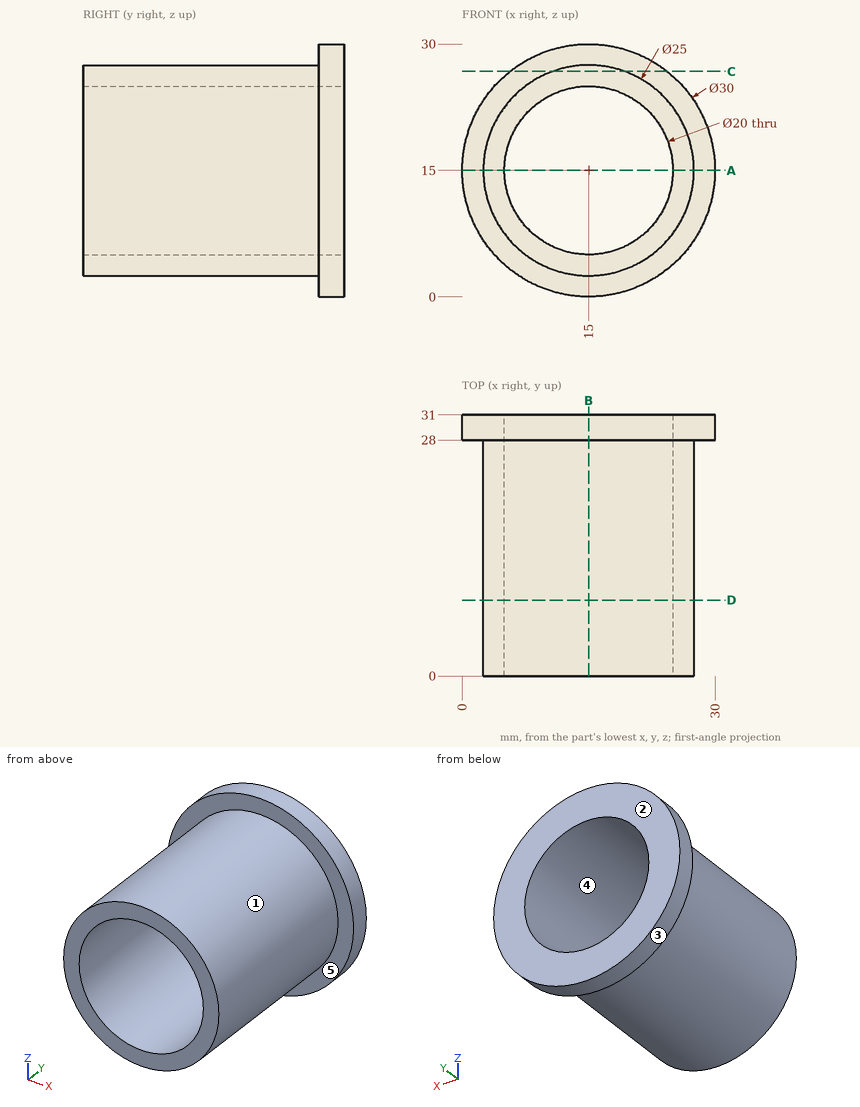
Answer from the drawing. Dimensions are ordinates in mm from the lowest x, y and z of the part. A direction names the side the tool comes from. Round coordinates to 2 decimals unless told otherwise and drop trailing zeros. Loops run counter-clockwise (first coordinate to the right, second up) from the corner with the lowest first, then second, coordinate; pieces in that order, holes last.
Q1. Section B-B on x = 15 is taken. Write down the section's boundary in (y, z), and give its area (3 significant figures).
Q2. Section D-D on y = 9 is taken. Write down the section's boundary in (x, z), and give its area (3 significant figures).
Q3. Section A-A on z = 15 is taken. Write down the section's boundary in (x, y).
Q4. Section C-C on z = 26.75 is taken. Write down the section's boundary in (x, y), and give its area (3 significant figures).
Q5. Which of the six approach directions +Z, -Z, +X, -X, +Y, -Y give full straight-line access (tool end or side, diameter ignored) to the marked faces 1 and 2?
Q6. Determine the mould class of the marked faces 3, 4 and 5 for opening direction Z: released by +Z, released by -Z, zero draft, split by the parting line, or undercut.
Q7. Consider probe 1 along Z at (x, y) = (15, 8.5); probe 2 along Y at (x, z) = (21.25, 2.5); probe 3 along X at (y, z) = (28.5, 21.75). Determine where each line is inside the solid, lowest interval first.
Q8. Each of these flat-tipped pins is pushed along its axis until it touches: pin 1 (10 mm diameter, centred on x = 21, y = 26.5, fed in from -Z); pin 2 (10 mm diameter, centred on y = 10.5, z = 9, fed in from -X); pin 3 (1.5 mm diameter, centred on y = 17, z = 6.5, fed in from -X); pin 4 (6 mm diameter, centred on x = 18.5, z = 23.5, fed in from -Y). Where does it stop, or does it pass through?
Output:
1. outline: (0, 2.5) - (28, 2.5) - (28, 0) - (31, 0) - (31, 5) - (0, 5) - close; (0, 25) - (31, 25) - (31, 30) - (28, 30) - (28, 27.5) - (0, 27.5) - close
1. area: 170 mm2
2. outline: circle Ø25 at (15, 15); hole circle Ø20 at (15, 15)
2. area: 177 mm2
3. outline: (0, 28) - (2.5, 28) - (2.5, 0) - (5, 0) - (5, 31) - (0, 31) - close; (25, 0) - (27.5, 0) - (27.5, 28) - (30, 28) - (30, 31) - (25, 31) - close
4. outline: (5.68, 28) - (10.74, 28) - (10.74, 0) - (19.26, 0) - (19.26, 28) - (24.32, 28) - (24.32, 31) - (5.68, 31) - close
4. area: 295 mm2
5. face 1: -Y
5. face 2: +Z, -Z, +X, -X, +Y
6. face 3: split by the parting line
6. face 4: undercut
6. face 5: zero draft
7. probe 1: z = 2.5 to 5, 25 to 27.5
7. probe 2: y = 28 to 31
7. probe 3: x = 1.6 to 7.62, 22.38 to 28.4
8. pin 1: stops at z = 0.05
8. pin 2: stops at x = 2.54
8. pin 3: stops at x = 5.19
8. pin 4: stops at y = 0
